Drawing for the job (mm, zero at the part's lowest x, y, z). A direction names the side the tool comes from. Give positions to 0.01 mm unless a question says otherwise; leave off trailing zeros. Order: outer loops, then holes, each group sorted by start corner. A loop starts at its lowest first (then second) coordinate and runs counter-clockwise, first axis right, second up. Notation, with made-up numbers: (-26.75, 74) -> (-0.75, 74) arc R20 cw to (-0.75, 93) -> close; hole circle Ø10 at (21.5, -17.75). An arc over 180 degrees is marked (long way). Use one line per item in the form item = value. Start each with the question number.
1) Cut at A-A, the plane y = 44.45. Give the cut face in (x, z).
2) Mould opens along Y. For the marked faces 1, 2, 3 and 4 say: pulls with the +Y half, pulls with the -Y half, needs draft (parallel to the pull), parting line crosses it, or undercut.
3) Cut at B-B, the plane z = 15.5. Give the cut face in (x, y), and give its area (3 significant figures).
4) Cut at D-D, the plane x = 133.5. Give the cut face in (y, z), and give its area (3 significant figures).
5) Probe line 1 (X direction, y = 44.45, z = 35); line 2 (X direction, y = 35.5, z = 23.5) (1 decimal); line 3 (Y direction, x = 28, z = 12). List the from-to ranges inside material, lowest first.
6) Cut at C-C, the plane x = 16. Give the cut face in (y, z), and give its area (3 significant figures).
7) Drop flat-ended pins along their axis: P1, Ø15, axis at x = 86.5, y = 77.5, coming from the +Z side; P2, Ø15, axis at x = 67.5, y = 35, coming from the -Z side; P3, Ø10, axis at x = 67.5, z = 37.5, coming from the +Y side. Give the stop position or say it passes through.
8) Tool access for the marked faces 5, 6 and 7: list every direction of +Z, -Z, +X, -X, +Y, -Y with a clear straight run to the whole face (end or side of a thin tool).
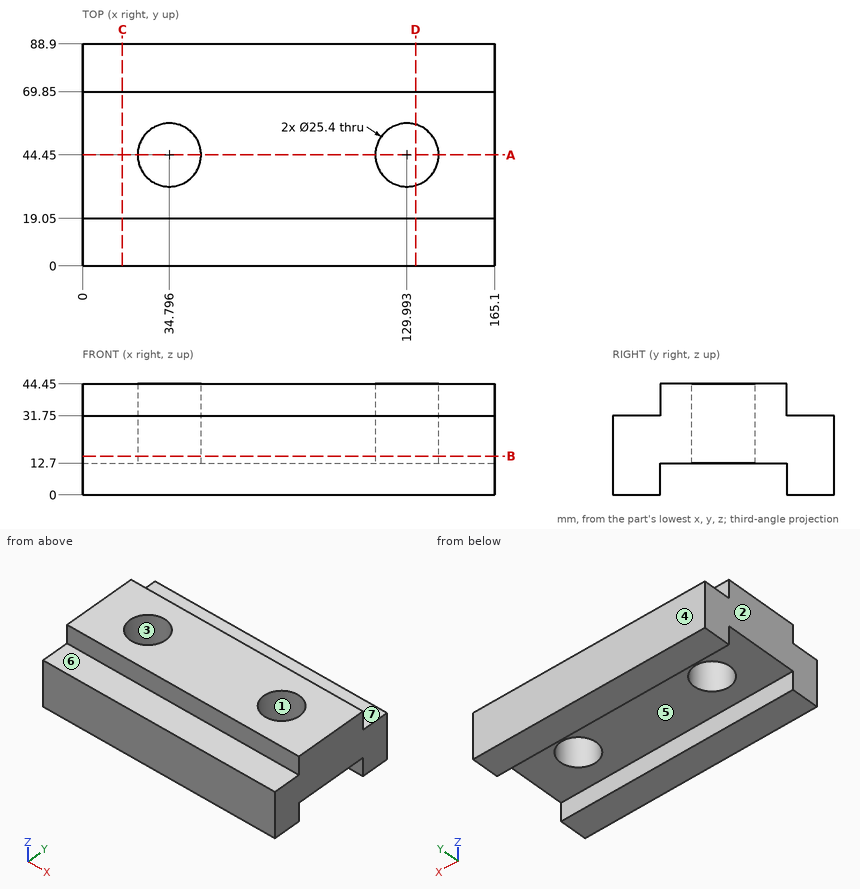
Result:
q1.outline = (0, 12.7) -> (22.1, 12.7) -> (22.1, 44.45) -> (0, 44.45) -> close; (47.5, 12.7) -> (117.29, 12.7) -> (117.29, 44.45) -> (47.5, 44.45) -> close; (142.69, 12.7) -> (165.1, 12.7) -> (165.1, 44.45) -> (142.69, 44.45) -> close
q2.face_1 = undercut
q2.face_2 = needs draft
q2.face_3 = undercut
q2.face_4 = pulls with the +Y half
q3.outline = (0, 0) -> (165.1, 0) -> (165.1, 88.9) -> (0, 88.9) -> close; hole circle Ø25.4 at (34.8, 44.45); hole circle Ø25.4 at (129.99, 44.45)
q3.area = 13,700 mm²
q4.outline = (0, 0) -> (19.05, 0) -> (19.05, 12.7) -> (32.24, 12.7) -> (32.24, 44.45) -> (19.05, 44.45) -> (19.05, 31.75) -> (0, 31.75) -> close; (56.66, 12.7) -> (69.85, 12.7) -> (69.85, 0) -> (88.9, 0) -> (88.9, 31.75) -> (69.85, 31.75) -> (69.85, 44.45) -> (56.66, 44.45) -> close
q4.area = 2,050 mm²
q5.line_1 = 0 to 22.1, 47.5 to 117.29, 142.69 to 165.1
q5.line_2 = 0 to 25.8, 43.8 to 121, 139 to 165.1
q5.line_3 = 0 to 19.05, 69.85 to 88.9
q6.outline = (0, 0) -> (19.05, 0) -> (19.05, 12.7) -> (69.85, 12.7) -> (69.85, 0) -> (88.9, 0) -> (88.9, 31.75) -> (69.85, 31.75) -> (69.85, 44.45) -> (19.05, 44.45) -> (19.05, 31.75) -> (0, 31.75) -> close
q6.area = 2,820 mm²
q7.P1 = 31.75
q7.P2 = 12.7
q7.P3 = 69.85
q8.face_5 = -Z, +X, -X
q8.face_6 = +Z, +X, -X, -Y
q8.face_7 = +Z, +X, -X, +Y
